from build123d import *

# Parameters (mm, degrees)
F0_W     = 24.4336966982
F0_H     = 23.368
F0_W_2   = 9.525
F0_H_2   = 9.525
F1_DEPTH = 6.35
F3_R     = 1.27
F4_DEPTH = 6.35


with BuildPart() as f1:
    # F0 (on Top) → F1 (new body)
    with BuildSketch(Plane.XY):
        Rectangle(F0_W, F0_H)
        Rectangle(F0_W_2, F0_H_2, mode=Mode.SUBTRACT)
    extrude(amount=F1_DEPTH)

    # F3
    f3_edges = [f1.edges().sort_by_distance(p)[0] for p in [
        (12.216848, 11.684, 3.175),
        (-12.216848, 11.684, 3.175),
        (-12.216848, -11.684, 3.175),
        (12.216848, -11.684, 3.175),
    ]]
    fillet(f3_edges, radius=F3_R)

    # F2 (on face) → F4 (cut)
    with BuildSketch(Plane.XY.offset(6.35)):
        with BuildLine():
            Line((-8.6625, 8.95), (-5.8625, 8.95))
            ThreePointArc((-5.8625, 8.95), (-7.2625, 10.35), (-8.6625, 8.95))
        make_face()
        with BuildLine():
            ThreePointArc((-8.6625, 8.95), (-7.2625, 7.55), (-5.8625, 8.95))
            Line((-5.8625, 8.95), (-8.6625, 8.95))
        make_face()
        with BuildLine():
            Line((5.8625, 8.95), (8.6625, 8.95))
            ThreePointArc((8.6625, 8.95), (7.2625, 10.35), (5.8625, 8.95))
        make_face()
        with BuildLine():
            ThreePointArc((5.8625, 8.95), (7.2625, 7.55), (8.6625, 8.95))
            Line((8.6625, 8.95), (5.8625, 8.95))
        make_face()
        with BuildLine():
            Line((5.8625, -8.95), (8.6625, -8.95))
            ThreePointArc((8.6625, -8.95), (7.2625, -7.55), (5.8625, -8.95))
        make_face()
        with BuildLine():
            ThreePointArc((5.8625, -8.95), (7.2625, -10.35), (8.6625, -8.95))
            Line((8.6625, -8.95), (5.8625, -8.95))
        make_face()
        with BuildLine():
            Line((-8.6625, -8.95), (-5.8625, -8.95))
            ThreePointArc((-5.8625, -8.95), (-7.2625, -7.55), (-8.6625, -8.95))
        make_face()
        with BuildLine():
            ThreePointArc((-8.6625, -8.95), (-7.2625, -10.35), (-5.8625, -8.95))
            Line((-5.8625, -8.95), (-8.6625, -8.95))
        make_face()
    extrude(amount=-F4_DEPTH, mode=Mode.SUBTRACT)


solid = f1.part
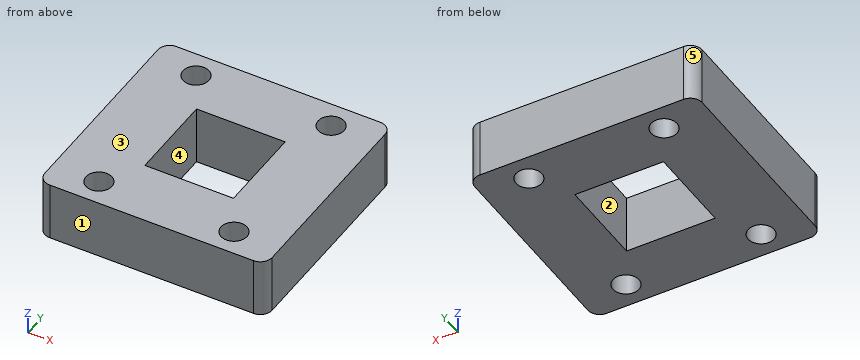
Read the model definition and answer for the solid it produces. Units are mm, in the model's axes. Face numbers are marked on the shaded views. A direction names the side the tool comes from. Coordinates: 2 decimals unless noted, no trailing zeros. Loops run counter-clockwise (first coordinate to the right, second up) from the corner with the lowest first, then second, coordinate; pieces in that order, holes last. Notation, with made-up numbers: (11, -34) - (68, -34) arc R23 cw to (68, -1) - close; hole circle Ø9 at (73.25, -38.5). An arc over 180 degrees is marked (long way). Answer in a Markdown table with one row per item.
Q1. The mould has two halves that part along Y. Classify the marked faces 1, 2 and 3: pulls with the +Y half, pulls with the -Y half, needs draft (parallel to the pull), parting line crosses it, or undercut.
Here are the results:
| item | result |
|---|---|
| face 1 | pulls with the -Y half |
| face 2 | undercut |
| face 3 | needs draft |
Q2. For the marked faces 4 and 5, determine the directions among +Z, -Z, +X, -X, +Y, -Y from which every point of the face is accessible in a straight line to the end or side of a thin tool.
Here are the results:
| item | result |
|---|---|
| face 4 | +Z, -Z |
| face 5 | +Z, -Z, -X, +Y |
Q3. Find section C-C on y = -8.95. Write down the section's boundary in (x, z).
Here are the results:
| item | result |
|---|---|
| outline | (-12.22, 0) - (-8.66, 0) - (-8.66, 6.35) - (-12.22, 6.35) - close; (-5.86, 0) - (5.86, 0) - (5.86, 6.35) - (-5.86, 6.35) - close; (8.66, 0) - (12.22, 0) - (12.22, 6.35) - (8.66, 6.35) - close |
Q4. Find section B-B on z = 5.75. Write down the section's boundary in (x, y), plus the area to 3 significant figures.
Here are the results:
| item | result |
|---|---|
| outline | (-12.22, -10.41) arc R1.27 ccw to (-10.95, -11.68) - (10.95, -11.68) arc R1.27 ccw to (12.22, -10.41) - (12.22, 10.41) arc R1.27 ccw to (10.95, 11.68) - (-10.95, 11.68) arc R1.27 ccw to (-12.22, 10.41) - close; hole circle Ø2.8 at (-7.26, -8.95); hole circle Ø2.8 at (-7.26, 8.95); hole (-4.76, -4.76) - (4.76, -4.76) - (4.76, 4.76) - (-4.76, 4.76) - close; hole circle Ø2.8 at (7.26, -8.95); hole circle Ø2.8 at (7.26, 8.95) |
| area | 454 mm^2 |
Q5. Find section A-A on y = -1.75. Write down the section's boundary in (x, z).
Here are the results:
| item | result |
|---|---|
| outline | (-12.22, 0) - (-4.76, 0) - (-4.76, 6.35) - (-12.22, 6.35) - close; (4.76, 0) - (12.22, 0) - (12.22, 6.35) - (4.76, 6.35) - close |
Q6. Straight lines are drawn through the part: line 1 along X through (y, z) = (-8.95, 3); line 2 along Y through (x, z) = (2, 2.5); line 3 along X through (y, z) = (2, 5.75). For each, find the intervals that lie inside material, in ascending order. Write a range as [from, to].
Here are the results:
| item | result |
|---|---|
| line 1 | x = [-12.22, -8.66], [-5.86, 5.86], [8.66, 12.22] |
| line 2 | y = [-11.68, -4.76], [4.76, 11.68] |
| line 3 | x = [-12.22, -4.76], [4.76, 12.22] |
